```python
from build123d import *

# Parameters (mm, degrees)
SALIENTE_EXTRUIR1_DEPTH = 4
CORTAR_EXTRUIR4_DEPTH   = 5
CROQUIS10_R             = 1.5
CORTAR_EXTRUIR5_DEPTH   = 5
CROQUIS12_R             = 2.575
CORTAR_EXTRUIR6_DEPTH   = 5
CROQUIS13_R             = 3
CORTAR_EXTRUIR7_DEPTH   = 2


with BuildPart() as part:
    # Croquis1 → Saliente-Extruir1 (new body)
    with BuildSketch(Plane(origin=(0, 0, 0), x_dir=(1, 0, 0), z_dir=(0, 1, 0))):
        with BuildLine():
            Line((-2.5, -25), (2.5, -25))
            ThreePointArc((2.5, -25), (6.035533906, -23.535533906), (7.5, -20))
            Line((7.5, -20), (7.5, -14))
            Line((7.5, -14), (13.5, -14))
            Line((13.5, -14), (13.5, -8))
            Line((13.5, -8), (7.5, -8))
            Line((7.5, -8), (7.5, -1.55))
            Line((7.5, -1.55), (5.45, -1.55))
            Line((5.45, -1.55), (5.45, -2.8))
            Line((5.45, -2.8), (2.55, -2.8))
            Line((2.55, -2.8), (2.55, -1.55))
            Line((2.55, -1.55), (0.5, -1.55))
            Line((0.5, -1.55), (0.5, 1.55))
            Line((0.5, 1.55), (2.55, 1.55))
            Line((2.55, 1.55), (2.55, 2.8))
            Line((2.55, 2.8), (5.45, 2.8))
            Line((5.45, 2.8), (5.45, 1.55))
            Line((5.45, 1.55), (7.5, 1.55))
            Line((7.5, 1.55), (7.5, 8))
            Line((7.5, 8), (13.5, 8))
            Line((13.5, 8), (13.5, 14))
            Line((13.5, 14), (7.5, 14))
            Line((7.5, 14), (7.5, 20))
            ThreePointArc((7.5, 20), (6.035533906, 23.535533906), (2.5, 25))
            Line((2.5, 25), (-2.5, 25))
            ThreePointArc((-2.5, 25), (-6.035533906, 23.535533906), (-7.5, 20))
            Line((-7.5, 20), (-7.5, -20))
            ThreePointArc((-7.5, -20), (-6.035533906, -23.535533906), (-2.5, -25))
        make_face()
    extrude(amount=SALIENTE_EXTRUIR1_DEPTH)

    # Croquis7 → Cortar-Extruir4 (cut, through all)
    with BuildSketch(Plane(origin=(0, 4, 0), x_dir=(1, 0, 0), z_dir=(0, 1, 0))):
        with BuildLine():
            Line((5.877341989, 1.55), (7.5, 1.55))
            Line((7.5, 1.55), (7.5, -1.55))
            Line((7.5, -1.55), (5.877341989, -1.55))
            ThreePointArc((5.877341989, -1.55), (5.375478098, -2.869619136), (4, -3.187930349))
            ThreePointArc((4, -3.187930349), (2.755747615, -2.971867524), (2.117475162, -1.882163243))
            ThreePointArc((2.117475162, -1.882163243), (0.52576038, -1.575149398), (0.14272275, 0))
            ThreePointArc((0.14272275, 0), (0.52576038, 1.575149398), (2.117475162, 1.882163243))
            ThreePointArc((2.117475162, 1.882163243), (2.755747615, 2.971867524), (4, 3.187930349))
            ThreePointArc((4, 3.187930349), (5.375478098, 2.869619136), (5.877341989, 1.55))
        make_face()
    extrude(amount=-CORTAR_EXTRUIR4_DEPTH, mode=Mode.SUBTRACT)

    # Croquis10 → Cortar-Extruir5 (cut, through all)
    with BuildSketch(Plane(origin=(0, 4, 0), x_dir=(1, 0, 0), z_dir=(0, 1, 0))):
        with Locations((8.560660172, 15.060660172)):
            Circle(CROQUIS10_R)
        with Locations((8.560660172, 6.939339828)):
            Circle(CROQUIS10_R)
        with Locations((8.560660172, -15.060660172)):
            Circle(CROQUIS10_R)
        with Locations((8.560660172, -6.939339828)):
            Circle(CROQUIS10_R)
    extrude(amount=-CORTAR_EXTRUIR5_DEPTH, mode=Mode.SUBTRACT)

    # Croquis12 → Cortar-Extruir6 (cut, through all)
    with BuildSketch(Plane.XZ):
        with Locations((0.5, -11.5)):
            Circle(CROQUIS12_R)
        with Locations((0.5, -19.5)):
            Circle(CROQUIS12_R)
    cortar_extruir6 = extrude(amount=-CORTAR_EXTRUIR6_DEPTH, mode=Mode.SUBTRACT)

    # Croquis13 → Cortar-Extruir7 (cut)
    with BuildSketch(Plane.XZ):
        with Locations((0.5, -11.5)):
            Circle(CROQUIS13_R)
        with Locations((0.5, -19.5)):
            Circle(CROQUIS13_R)
    cortar_extruir7 = extrude(amount=-CORTAR_EXTRUIR7_DEPTH, mode=Mode.SUBTRACT)

    # Simetría1: Cortar-Extruir6, Cortar-Extruir7 across plane
    add(cortar_extruir6.mirror(Plane.XY), mode=Mode.SUBTRACT)
    add(cortar_extruir7.mirror(Plane.XY), mode=Mode.SUBTRACT)


solid = part.part
```
Geometry: final body of the model. Coordinates: model frame, mm. A direction names the side the tool comes from. Round coordinates to 2 decimals unless told otherwise and drop trailing zeros. Order: outer loops, then holes, each group sorted by start corner. A loop starts at its lowest first (then second) coordinate and runs counter-clockwise, first axis right, second up. Notation, with made-up numbers: (17.5, -11.75) - (66.5, -11.75) arc R36 ccw to (66.5, 24.25) - close; hole circle Ø11 at (-24, 53). An arc over 180 degrees is marked (long way). Use CSV: the item, a comma, the result in double quotes. Start each with the question number.
Q1. Section query C-C (z = -19.5). Return loops of the section in (x, y) (3 decimals), and give its area (3 significant figures).
Q2. Mould query, pull axis Z, two halves, no side actions, for faces 5 (the face through (12, 2, -14)), 6 (the face through (13.5, 2, 11)), 7 (the face through (-0.15, 0.99, -22.43)). Classes: +Z half, -Z half, draft (parallel to the pull), parting line (faces both ways), or undercut.
Q3. Section query B-B (z = 11.5). Return loops of the section in (x, y) (3 decimals).
Q4. Section query D-D (y = 0.5). State how many separate pieces and enclosed holes the cut face has, and give its area (3 significant figures).
Q5. Material intervals for line 1 along Z through (x, y) = (0.5, 1.3); line 2 along X through (y, z) = (1.25, 11.5); line 3 along Z through (x, y) = (0.5, 2.85) (3 decimals), sorted ascending. Write a range as from..to.
Q6. Access query for faces 1 (the face through (12, 2, 8)), 2 (the face through (-0.15, 0.99, 22.43)), 3 (the face through (5.36, 2.028, -2.883)), 4 (the face through (6, 1.97, 23.57)). Directions: +Z, -Z, +X, -X, +Y, -Y. A direction counts if a zero-diameter tool reaches every point of the face in a straight line with its end or side. Return the directions, or none.
Q7. First-contact query: pin 1 (1.2 mm diameter, centred on x = 11.5, y = 1.5, fed in from +Z); pin 2 (1.9 mm diameter, centred on x = 12, y = 1, fed in from -Z); pin 3 (3 mm diameter, centred on x = 0.5, z = -11, fed in from -Y); pin 4 (1.2 mm diameter, centred on y = 3, z = -5, fed in from +X). Flat tips, straight axial feed; report the tip coordinate or a pass-through.
Q8. Section query A-A (x = 10.5). Return loops of the section in (y, z), and give its area (3 significant figures).
Result set:
1,outline,"(-7.5, 0) - (-2.5, 0) - (-2.5, 2) - (-2.075, 2) - (-2.075, 4) - (-7.5, 4) - close; (3.075, 2) - (3.5, 2) - (3.5, 0) - (7.5, 0) - (7.5, 4) - (3.075, 4) - close"
1,area,"37.7 mm2"
2,face 5,"-Z half"
2,face 6,"draft"
2,face 7,"undercut"
3,outline,"(-7.5, 0) - (-2.5, 0) - (-2.5, 2) - (-2.075, 2) - (-2.075, 4) - (-7.5, 4) - close; (3.075, 2) - (3.5, 2) - (3.5, 0) - (13.5, 0) - (13.5, 4) - (3.075, 4) - close"
4,separate pieces,"1"
4,enclosed holes,"4"
4,area,"648 mm2"
5,line 1,"z = -25..-22.5, -16.5..-14.5, -8.5..-1.55, 1.55..8.5, 14.5..16.5, 22.5..25"
5,line 2,"x = -7.5..-2.5, 3.5..13.5"
5,line 3,"z = -25..-22.075, -16.925..-14.075, -8.925..-1.55, 1.55..8.925, 14.075..16.925, 22.075..25"
6,face 1,"+X, +Y, -Y"
6,face 2,"-Y"
6,face 3,"+Y, -Y"
6,face 4,"+Z, +X, +Y, -Y"
7,pin 1,"stops at z = 14"
7,pin 2,"stops at z = -14"
7,pin 3,"passes through"
7,pin 4,"stops at x = 7.5"
8,outline,"(0, -14) - (4, -14) - (4, -8) - (0, -8) - close; (0, 8) - (4, 8) - (4, 14) - (0, 14) - close"
8,area,"48.0 mm2"
